Part model, mm, in its own coordinate system. Face numbers are marked on the shaded views. A direction names the side the tool comes from. Give positions to 0.01 mm unless a question says otherwise; leave off trailing zeros. Loops run counter-clockwise (first coordinate to the right, second up) from the corner with the lowest first, then second, coordinate; pieces in that order, holes last. Notation, with made-up numbers: M 55,4.5 L 92,4.5 A27 ccw 92,33.5 Z; hole C 44.25,-2.5 d6. An arc over 180 degrees is marked long. Put each result on its own line as item: value. Start each with the question number.
Autodesk Inventor part; units mm, degrees
ref_plane "YZ Plane" through (0, 0, 0) normal (1, 0, 0) x (0, 1, 0)
ref_plane "XZ Plane" through (0, 0, 0) normal (0, 1, 0) x (-1, 0, 0)
ref_plane "XY Plane" through (0, 0, 0) normal (0, 0, 1) x (1, 0, 0)
sketch "Sketch1" plane through (0, 0, 0) normal (0, 1, 0) x (-1, 0, 0)
  line L0 (15, 14.965) -> (-15, 14.965)
  line L1 (-15, 14.965) -> (-15, -14.965)
  line L2 (-15, -14.965) -> (15, -14.965)
  line L3 (15, -14.965) -> (15, 14.965)
  point P0 (0, 0)
  dimension "d0" = 29.93
  dimension "d1" = 30
  dimension "d2" = 15
  dimension "d3" = 14.965
extrude "Plate1" add sketch "Sketch1" along normal blind 1.5
sketch "Sketch2" plane through (-15, 0, -13.465) normal (0, 0, -1) x (-1, 0, 0)
  line L0 (-30, 0) -> (0, 0)
  line L1 (0, 0) -> (0, 32)
  line L2 (0, 32) -> (-30, 32)
  line L3 (-30, 32) -> (-30, 0)
edge flange "Flange1" height 32 angle 90 thickness 1.5 bend radius 0.31 thickness toward (0, 0, -1) relief tear relief width 1.5 relief depth 0.75 corner gap 0.31 corner form 0 edges at (0, 1.5, -14.965) (0, 1.5, 14.965) wall of the first edge with corners at (15, 0, -13.465) (-15, 0, -13.465) (-15, 32, -13.465) (15, 32, -13.465)
bend "Bend1"
corner "Corner1"
sketch "Sketch3" plane through (-15, 32, 14.965) normal (0, 0, 1) x (1, 0, 0)
  line L0 (0, 0) -> (30, 0)
  line L1 (0, -30.19) -> (0, 0)
  circle A0 centre (15, -10) radius 10
  line L2 (0, -18.5) -> (30, -18.5)
  line L3 (30, -18.5) -> (30, -28.5)
  line L4 (30, -28.5) -> (0, -28.5)
  line L5 (0, -28.5) -> (0, -18.5)
  line L6 (30, -18.5) -> (24.0624, -5.7723)
  line L7 (0, -18.5) -> (5.9376, -5.7723)
  line L8 (0, 0) -> (30, 0)
  line L9 (30, 0) -> (30, -25)
  line L10 (30, -25) -> (0, -25)
  line L11 (0, -25) -> (0, 0)
  point P0 (15, -32)
  point P1 (15, 0)
  dimension "d15" = 10
  dimension "d16" = 0
  dimension "d17" = 20
  dimension "d18" = 8.5
  dimension "d19" = 0
  dimension "d20" = 30
  dimension "d21" = 10
  dimension "d22" = 25
extrude "Extrusion1" cut sketch "Sketch3" against normal blind 35 contours L0 A0 L7 L1 | L0 L9 L6 A0
sketch "Sketch4" plane through (15, 1.81, -14.965) normal (0, 0, -1) x (-1, 0, 0)
  arc A0 (24.0624, 24.4177) -> (5.9376, 24.4177) centre (15, 20.19) ccw
  circle A1 centre (15, 20.19) radius 2.6
  circle A2 centre (8, 20.19) radius 1.05
  circle A3 centre (22, 20.19) radius 1.05
  circle A4 centre (15, 27.19) radius 1.05
  circle A5 centre (15, 13.19) radius 1.05
  point P0 (15, -1.81)
  dimension "d25" = 5.2
  dimension "d26" = 0
  dimension "d27" = 7
  dimension "d28" = 2.1
  dimension "d29" = 7
  dimension "d30" = 0
  dimension "d31" = 2.1
  dimension "d32" = 0
  dimension "d33" = 7
  dimension "d34" = 2.1
  dimension "d35" = 7
  dimension "d36" = 0
  dimension "d37" = 2.1
extrude "Extrusion2" cut sketch "Sketch4" against normal blind 1.5
sketch "Sketch5" plane through (-15, 1.81, 14.965) normal (0, 0, 1) x (1, 0, 0)
  arc A0 (24.0624, 24.4177) -> (5.9376, 24.4177) centre (15, 20.19) ccw
  circle A1 centre (15, 20.19) radius 1.5
  point P0 (15, -1.81)
  dimension "d40" = 3
extrude "Extrusion3" cut sketch "Sketch5" against normal blind 1.5
equation "\"d4\" = Thickness"
equation "\"d5\" = BendReliefWidth"
equation "\"d6\" = BendReliefDepth"
equation "\"d7\" = MinimumRemnant"
equation "\"d8\" = TransitionRadius"
equation "\"d11\" = BendRadius"
equation "\"d12\" = CornerReliefSize"
equation "\"d13\" = GapSize"
equation "\"d14\" = JacobiRadiusSize"
equation "\"BendReliefWidth\" = Thickness"
equation "\"BendReliefDepth\" = 0.5 * Thickness"
equation "\"CornerReliefSize\" = 4 * Thickness"
equation "\"MinimumRemnant\" = 2 * Thickness"
equation "\"TransitionRadius\" = BendRadius"
equation "\"JacobiRadiusSize\" = BendRadius"
equation "\"GapSize\" = Thickness"
properties part number "partpart" material "Aluminum 6061-AHC"
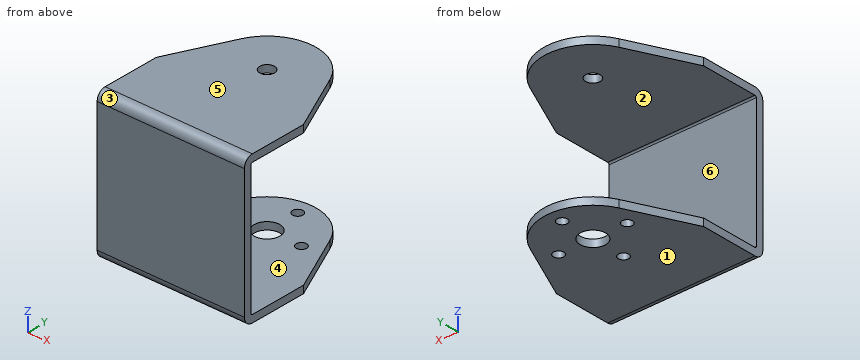
1) Pin check, flat tips, straight feed: pin 1 Ø3 at (x, z) = (-1, 1) entering from +Y; pin 2 Ø10 at (y, z) = (8.5, -1.5) entering from -X. Stop position of each tip, or through.
2) Band-saw the part on D-D on x = -7. Give the cut face in (y, z) (3 decimals).
3) Band-saw the part on A-A on y = 10.5. Give the cut face in (x, z) (3 decimals), then the cut area to 3 significant figures.
4) Wall check: L1, parallel to Z at x = -2.75, y = 20 (3 decimals); L2, parallel to Y at x = -7, z = -14.05; L3, parallel to Y at x = 1.5, z = -10.5. Give the ranges that are in metal, low to high.
5) Mould opens along Z. For the marked faces 1, 2, 3 and 4 say: +Z half, -Z half, draft (parallel to the pull), parting line (faces both ways), or undercut.
6) Band-saw the part on C-C on y = 29. Give the cut face in (x, z) (3 decimals), then the cut area to 3 significant figures.
7) Which spindle directions (+Z, -Z, +X, -X, +Y, -Y) get a long thin tool onto all of the face, cutting with end or side? Do the marked faces 5 and 6. Say none if no direction does.
8) Band-saw the part on B-B on x = 0. Give the cut face in (y, z) (3 decimals).
Evaluation:
1. pin 1: y = 1.5
1. pin 2: through
2. outline: M 0,-13.155 A1.81 ccw 1.81,-14.965 L 20.95,-14.965 L 20.95,-13.465 L 1.81,-13.465 A0.31 cw 1.5,-13.155 L 1.5,13.155 A0.31 cw 1.81,13.465 L 29.141,13.465 L 29.141,14.965 L 1.81,14.965 A1.81 ccw 0,13.155 Z; M 23.05,-14.965 L 29.141,-14.965 L 29.141,-13.465 L 23.05,-13.465 Z
3. outline: M -15,-14.965 L 15,-14.965 L 15,-13.465 L -15,-13.465 Z; M -15,13.465 L 15,13.465 L 15,14.965 L -15,14.965 Z
3. area: 90.0 mm2
4. L1: -14.965 to -13.465, 13.465 to 14.965
4. L2: 0.24 to 20.95, 23.05 to 29.14
4. L3: 0 to 1.5
5. face 1: -Z half
5. face 2: undercut
5. face 3: +Z half
5. face 4: undercut
6. outline: M -7.141,-14.965 L -1.05,-14.965 L -1.05,-13.465 L -7.141,-13.465 Z; M -7.141,13.465 L 7.141,13.465 L 7.141,14.965 L -7.141,14.965 Z; M 1.05,-14.965 L 7.141,-14.965 L 7.141,-13.465 L 1.05,-13.465 Z
6. area: 39.7 mm2
7. face 5: +Z, +X, -X, +Y, -Y
7. face 6: +X, -X, +Y
8. outline: M 0,-13.155 A1.81 ccw 1.81,-14.965 L 13.95,-14.965 L 13.95,-13.465 L 1.81,-13.465 A0.31 cw 1.5,-13.155 L 1.5,13.155 A0.31 cw 1.81,13.465 L 20.5,13.465 L 20.5,14.965 L 1.81,14.965 A1.81 ccw 0,13.155 Z; M 16.05,-14.965 L 19.4,-14.965 L 19.4,-13.465 L 16.05,-13.465 Z; M 23.5,13.465 L 32,13.465 L 32,14.965 L 23.5,14.965 Z; M 24.6,-14.965 L 27.95,-14.965 L 27.95,-13.465 L 24.6,-13.465 Z; M 30.05,-14.965 L 32,-14.965 L 32,-13.465 L 30.05,-13.465 Z
